Geometry check sheet. Reference: drawing and pictorial views, mm from the part's lowest x, y, z. Round coordinates to 2 decimals unless told otherwise and drop trailing zeros. Loops run counter-clockwise (first coordinate to the right, second up) from the corner with the lowest first, then second, coordinate; pieces in that order, holes last. Notation, with made-up numbers: M 25.5,-4.5 L 74.5,-4.5 A13 ccw 74.5,19.5 Z; hole C 15,-21.75 d11. An arc over 180 degrees is marked long. One line per question, with ' | ' between items. Start each with the question number.
(1) Section check B-B (y = 236). Record the boundary of the cut face in (x, z), and give its area (3 significant figures).
(2) Go/stop test with flat-tipped pins: P1, Ø8, axis at x = 20.5, y = 55.5, coming from the -Z side; P2, Ø8, axis at x = 33.5, y = 407.5, coming from the +Z side; P3, Ø2, axis at y = 95.5, z = 24, coming from the -X side; P4, Ø5, axis at x = 16, z = 16.5, coming from the -Y side. Record where each tip stops, or that it passes through.
(3) Section check A-A (z = 4). Record the boundary of the cut face in (x, y), and give its area (3 significant figures).
(4) Thickness scan on probe 1 along X at (y, z) = (407.5, 26); probe 2 along X at (y, z) = (407, 18); probe 3 along Y at (x, z) = (6.5, 13). Record the ranges inside material, lowest first. Write a range as [from, to].
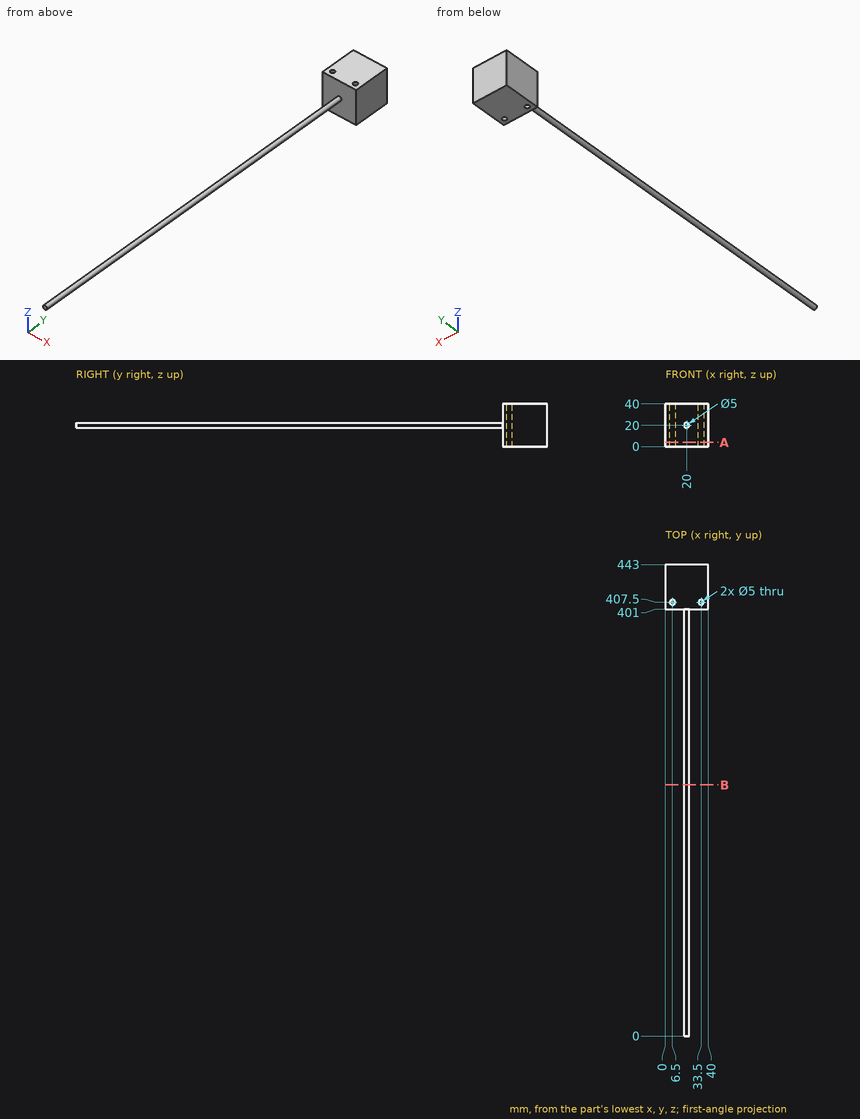
The answers:
1) outline: C 20,20 d5 | area: 19.6 mm²
2) P1: z = 17.5 | P2: z = 40 | P3: through | P4: y = 401
3) outline: M 0,401 L 40,401 L 40,443 L 0,443 Z; hole C 6.5,407.5 d5; hole C 33.5,407.5 d5 | area: 1,640 mm²
4) probe 1: [0, 4], [9, 31], [36, 40] | probe 2: [0, 4.05], [8.95, 31.05], [35.95, 40] | probe 3: [401, 405], [410, 443]
